Read the model definition and answer for the solid it produces. Units are mm, in the model's axes. A direction names the side the tool comes from. Round coordinates to 2 decimals unless told otherwise and drop trailing zeros. Write each loop counter-clockwise with the first axis right and the second up, starting at its lowest first coordinate (ties: lowest second). Pieces come first, ordered by that corner, then holes.
from build123d import *

# Parameters (mm, degrees)
SKETCH3_R   = 63.5
SKETCH3_R_2 = 51.1302


with BuildPart() as part:
    # Sketch1 → Revolve1 (revolve)
    with BuildSketch(Plane.XY, mode=Mode.PRIVATE) as revolve1_sk:
        Polygon((-110.49, -63.5), (-58.928, -63.5), (-58.928, -57.0357), (-110.49, -57.3786), align=None)
    revolve(revolve1_sk.sketch.rotate(Axis((-110.49, 0, 0), (1, 0, 0)), 270), axis=Axis((-110.49, 0, 0), (1, 0, 0)))


with BuildPart() as body_2:
    # Sketch2 → Revolve2 (revolve)
    with BuildSketch(Plane.XY, mode=Mode.PRIVATE) as revolve2_sk:
        Polygon((57.3786, 110.49), (57.0357, 58.928), (63.5, 58.928), (63.5, 110.49), align=None)
    revolve(revolve2_sk.sketch.rotate(Axis((0, 0, 0), (0, 1, 0)), 90), axis=Axis((0, 0, 0), (0, 1, 0)))


with BuildPart() as sweep1_tool:
    # Sweep1: sweep along a path in Sketch4
    with BuildLine(Plane.XY) as sweep1_path:
        ThreePointArc((-58.928, 0), (-17.259612, 17.259612), (0, 58.928))
    # Sketch3 → Sweep1 (sweep)
    with BuildSketch(Plane(origin=(-58.928, 0, 0), x_dir=(0, 0, -1), z_dir=(1, 0, 0))):
        Circle(SKETCH3_R)
        Circle(SKETCH3_R_2, mode=Mode.SUBTRACT)
    sweep(path=sweep1_path.line)


with BuildPart() as part_1:
    add(part.part)


with BuildPart() as part_2:
    # Sweep1: joined with sweep1_tool
    add(part_1.part.fuse(sweep1_tool.part, body_2.part, tol=0.00001))


solid = part_2.part
Q1. Determine the mould class of faces 1 (the conical face through (-17.183, 84.348, -54.563)), 2 (the flat face through (-110.49, 56, 14)), 3 (the cylindrical face through (61.99, 85.07, 13.77)) for opening direction Z: pulls with the +Z half, pulls with the -Z half, needs draft (parallel to the pull), parting line crosses it, or undercut.
Verdict:
face 1: undercut
face 2: needs draft
face 3: parting line crosses it
Q2. Section A-A (y = 79) is taken. Determine the outline of the cut face in (x, z).
Verdict:
outline: circle Ø127 at (0, 0); hole circle Ø114.34 at (0, 0)
Q3. A straight line is drawn through the part: probe 1 along X at (y, z) = (34.5, -43). Find the intervals that lie inside material, in ascending order.
Verdict:
probe 1: x = -58.93 to -39.42, 24.15 to 43.86
Q4. Flat-ended cylindrical pins translate along their axes: pin 1 Ø8 at (x, z) = (12.5, 6) entering from -Y; pin 2 Ø4 at (x, y) = (-60.5, 9) entering from -Z; pin 3 Ø6 at (y, z) = (-29, 27.5) entering from +X. Find the tip coordinate at first contact, or state that the pin passes through.
Verdict:
pin 1: stops at y = -42.95
pin 2: stops at z = -63.11
pin 3: stops at x = 20.92
Q5. Section B-B (x = -68.5) is taken. Determine the outline of the cut face in (y, z).
Verdict:
outline: circle Ø127 at (0, 0); hole circle Ø114.2 at (0, 0)
Q6. Which of the six approach directions +Z, -Z, +X, -X, +Y, -Y give full straight-line access (tool end or side, diameter ignored) to faces 4 (the flat face through (-21, 58.928, -47)), 5 (the flat face through (56, 110.49, 14)), 6 (the conical face through (-85.07, -2.515, -57.154))?
Verdict:
face 4: +Y
face 5: +Z, -Z, +X, -X, +Y
face 6: -X
